Verification items for the finished model (mm, model axes). Face numbers are marked on the shaded views. A direction names the side the tool comes from. Coordinates: 2 decimals unless noted, no trailing zeros. Order: outer loops, then holes, each group sorted by start corner. A loop starts at its lowest first (then second) coordinate and runs counter-clockwise, first axis right, second up. Notation, with made-up numbers: M 84.25,49 L 127.25,49 A14 cw 127.25,54 Z; hole C 33,35 d8. An arc over 180 degrees is marked long. Use one line per item in the form item = value. Start each with the question number.
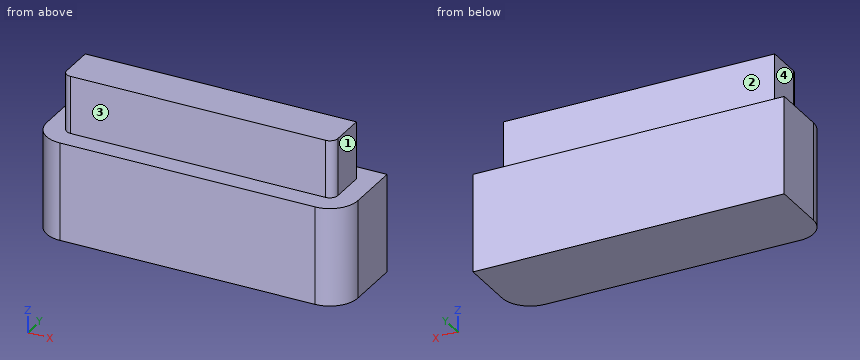
Autodesk Inventor part; units mm, degrees
ref_plane "YZ Plane" through (0, 0, 0) normal (1, 0, 0) x (0, 1, 0)
ref_plane "XZ Plane" through (0, 0, 0) normal (0, 1, 0) x (-1, 0, 0)
ref_plane "XY Plane" through (0, 0, 0) normal (0, 0, 1) x (1, 0, 0)
sketch "Sketch1" plane through (0, 0, 0) normal (0, 0, 1) x (1, 0, 0)
  line L0 (-22.25, 5.95) -> (22.25, 5.95) construction
  line L1 (22.25, 5.95) -> (22.25, -1.95)
  line L2 (18.25, -5.95) -> (-18.25, -5.95)
  line L3 (-22.25, -1.95) -> (-22.25, 5.95)
  line L4 (-22.25, 5.95) -> (22.25, -5.95) construction
  line L5 (22.25, 5.95) -> (-22.25, -5.95) construction
  arc A0 (-22.25, -1.95) -> (-18.25, -5.95) centre (-18.25, -1.95) ccw
  arc A1 (18.25, -5.95) -> (22.25, -1.95) centre (18.25, -1.95) ccw
  line L6 (-18.25, -5.95) -> (18.25, -5.95)
  line L7 (-22.25, -1.95) -> (-22.25, 5.95)
  line L8 (-22.25, 5.95) -> (22.25, 5.95)
  line L9 (22.25, 5.95) -> (22.25, -1.95)
  point P0 (0, 0)
  dimension "d0" = 44.5
  dimension "d1" = 11.9
  dimension "d2" = 4
extrude "Extrusion1" add sketch "Sketch1" along normal blind 14
sketch "Sketch2" plane through (0, 0, 14) normal (0, 0, 1) x (1, 0, 0)
  line L0 (-22.25, 5.95) -> (-22.25, -1.95)
  arc A0 (-22.25, -1.95) -> (-18.25, -5.95) centre (-18.25, -1.95) ccw
  line L1 (-18.25, -5.95) -> (18.25, -5.95)
  arc A1 (18.25, -5.95) -> (22.25, -1.95) centre (18.25, -1.95) ccw
  line L2 (22.25, -1.95) -> (22.25, 5.95)
  line L3 (22.25, 5.95) -> (-22.25, 5.95)
  line L4 (-19.3806, 3.0806) -> (-19.3806, -1.95)
  arc A2 (-19.3806, -1.95) -> (-18.25, -3.0806) centre (-18.25, -1.95) ccw
  line L5 (-18.25, -3.0806) -> (18.25, -3.0806)
  arc A3 (18.25, -3.0806) -> (19.3806, -1.95) centre (18.25, -1.95) ccw
  line L6 (19.3806, -1.95) -> (19.3806, 3.0806)
  line L7 (19.3806, 3.0806) -> (-19.3806, 3.0806)
  point P0 (0, 0)
extrude "Extrusion2" add sketch "Sketch2" along normal blind 8.2 contours L7 L6 A3 L5 A2 L4
sketch "Sketch3" plane through (0, 0, 0) normal (0, 0, -1) x (-1, 0, 0)
  point P0 (0, 0)
  point P1 (0, 0)
sketch "Sketch4" plane through (-22.25, 5.95, 0) normal (0, 1, 0) x (1, 0, 0)
  line L0 (44.5, 0) -> (0, 0) construction
  line L1 (0, 0) -> (0, -14) construction
  line L2 (44.5, -14) -> (0, -14) construction
  line L3 (44.5, 0) -> (44.5, -14) construction
  point P0 (22.25, 0)
  point P1 (22.25, -7)
properties part number "ps2conn" material "PET Plastic"
1. Material ranges on line 1 along Y through (x, z) = (14, 17); line 2 along X through (y, z) = (1.25, 15.25); line 3 along Z through (x, y) = (-1, 5), recorded low to high.
2. Tool access check on the marked faces 1, 2, 3 and 4. Record the directions out of +Z, -Z, +X, -X, +Y, -Y that give a thin tool (end or side, any length) a straight path to the whole face; none if there is none.
3. Cross-section at D-D on y = -5. Enter the section's corners in (x, z), and give its area (3 significant figures).
4. Cross-section at C-C on y = 4.5. Enter the section's corners in (x, z), and give its area (3 significant figures).
5. Depth check by flat-ended pin: P1, Ø2, axis at y = -3.5, z = 6.5, coming from the +X side; P2, Ø3, axis at x = -6.5, z = 16.5, coming from the +Y side; P3, Ø1.5, axis at y = 1.5, z = 18.5, coming from the +X side. Enter the tip coordinate at first touch or a pass-through.
6. Cross-section at A-A on x = 0. Enter the section's corners in (y, z), and give its area (3 significant figures).
7. Cross-section at B-B on z = 19. Enter the section's corners in (x, y), and give its area (3 significant figures).
Final values:
q1.line_1 = -3.08 to 3.08
q1.line_2 = -19.38 to 19.38
q1.line_3 = 0 to 14
q2.face_1 = +Z, +X, +Y, -Y
q2.face_2 = +Z, +X, -X, +Y
q2.face_3 = +Z, +X, -X, -Y
q2.face_4 = +Z, -X, +Y, -Y
q3.outline = M -20.84,0 L 20.84,0 L 20.84,14 L -20.84,14 Z
q3.area = 583 mm2
q4.outline = M -22.25,0 L 22.25,0 L 22.25,14 L -22.25,14 Z
q4.area = 623 mm2
q5.P1 = 22.21
q5.P2 = 3.08
q5.P3 = 19.38
q6.outline = M -5.95,0 L 5.95,0 L 5.95,14 L 3.08,14 L 3.08,22.2 L -3.08,22.2 L -3.08,14 L -5.95,14 Z
q6.area = 217 mm2
q7.outline = M -19.38,-1.95 A1.13 ccw -18.25,-3.08 L 18.25,-3.08 A1.13 ccw 19.38,-1.95 L 19.38,3.08 L -19.38,3.08 Z
q7.area = 238 mm2
